Design review of the part built by this model. Coordinates are the model's own, in mm. A direction names the side the tool comes from. Coordinates: 2 decimals unless noted, no trailing zeros. Order: outer loops, then holes, each group sorted by start corner. A loop starts at its lowest first (then second) coordinate and runs counter-clockwise, first axis right, second up. Notation, with made-up numbers: M 0.5,-30 L 31.5,-30 A28 cw 31.5,0 Z; hole C 42.5,-18.75 d4. An arc over 180 degrees is marked long. Answer as a JSON object with one key per item and string values.
from build123d import *

# Parameters (mm, degrees)
BOSS_EXTRUDE1_DEPTH = 8
SKETCH2_R           = 1.75
CUT_EXTRUDE1_DEPTH  = 4


with BuildPart() as part:
    # Sketch1 → Boss-Extrude1 (new body)
    with BuildSketch(Plane.XY):
        with BuildLine():
            Line((-21, 0), (-12, 0))
            ThreePointArc((-12, 0), (-10.585786438, 0.585786438), (-10, 2))
            Line((-10, 2), (-10, 6.5))
            Line((-10, 6.5), (10, 6.5))
            Line((10, 6.5), (10, 2))
            ThreePointArc((10, 2), (10.585786438, 0.585786438), (12, 0))
            Line((12, 0), (21, 0))
            Line((21, 0), (21, 3))
            Line((21, 3), (13, 3))
            Line((13, 3), (13, 7.5))
            ThreePointArc((13, 7.5), (12.414213562, 8.914213562), (11, 9.5))
            Line((11, 9.5), (-11, 9.5))
            ThreePointArc((-11, 9.5), (-12.414213562, 8.914213562), (-13, 7.5))
            Line((-13, 7.5), (-13, 3))
            Line((-13, 3), (-21, 3))
            Line((-21, 3), (-21, 0))
        make_face()
    extrude(amount=BOSS_EXTRUDE1_DEPTH)

    # Sketch2 → Cut-Extrude1 (cut, through all)
    with BuildSketch(Plane(origin=(0, 3, 0), x_dir=(1, 0, 0), z_dir=(0, 1, 0))):
        with Locations((-17, -4)):
            Circle(SKETCH2_R)
        with Locations((17, -4)):
            Circle(SKETCH2_R)
    extrude(amount=-CUT_EXTRUDE1_DEPTH, mode=Mode.SUBTRACT)


solid = part.part
1) Tool access review of faces 5 (the flat face through (13, 5, 4)), 6 (the flat face through (-13, 5, 4)), 7 (the flat face through (0, 6.5, 4)): name each direction out of +Z, -Z, +X, -X, +Y, -Y from which nothing blocks a thin tool from reaching the whole face with its end or side.
Taken from the geometry:
{"face 5": "+Z, -Z, +X, +Y", "face 6": "+Z, -Z, -X, +Y", "face 7": "+Z, -Z, -Y"}
2) Add section B-B (y = 6). State the section outline as (x, z) points, and give its area (3 significant figures).
Taken from the geometry:
{"outline": "M -13,0 L -10,0 L -10,8 L -13,8 Z; M 10,0 L 13,0 L 13,8 L 10,8 Z", "area": "48.0 mm2"}
3) Add section C-C (x = -17). State the section outline as (y, z) points, and give its area (3 significant figures).
Taken from the geometry:
{"outline": "M 0,0 L 3,0 L 3,2.25 L 0,2.25 Z; M 0,5.75 L 3,5.75 L 3,8 L 0,8 Z", "area": "13.5 mm2"}
4) Add section A-A (y = 2.5). State the section outline as (x, z) points, and give its area (3 significant figures).
Taken from the geometry:
{"outline": "M -21,0 L -10,0 L -10,8 L -21,8 Z; M 10,0 L 21,0 L 21,8 L 10,8 Z; hole C -17,4 d3.5; hole C 17,4 d3.5", "area": "157 mm2"}
5) Mouldability with a two-part tool opening along X and no side actions: class faces 1 (the flat face through (10, 4, 4)), 2 (the flat face through (17, 3, 2)), 3 (the flat face through (-21, 2, 4)), 4 (the cylindrical face through (10.57, 0.6, 3.94)) as released by +X, released by -X, zero draft, split by the parting line, or undercut.
Taken from the geometry:
{"face 1": "undercut", "face 2": "zero draft", "face 3": "released by -X", "face 4": "undercut"}
6) To check wall thickness, follow L1, parallel to X at y = 5.25, z = 2.5; L2, parallel to X at y = 2.05, z = 4; L3, parallel to X at y = 0.7, z = 4. State the ranges of each line that lie inside material, in increasing order.
Taken from the geometry:
{"L1": "x = -13 to -10, 10 to 13", "L2": "x = -21 to -18.75, -15.25 to -10, 10 to 15.25, 18.75 to 21", "L3": "x = -21 to -18.75, -15.25 to -10.48, 10.48 to 15.25, 18.75 to 21"}
7) Add section D-D (z = 4). State the section outline as (x, y) points, and give its area (3 significant figures).
Taken from the geometry:
{"outline": "M -21,0 L -18.75,0 L -18.75,3 L -21,3 Z; M -15.25,0 L -12,0 A2 ccw -10,2 L -10,6.5 L 10,6.5 L 10,2 A2 ccw 12,0 L 15.25,0 L 15.25,3 L 13,3 L 13,7.5 A2 ccw 11,9.5 L -11,9.5 A2 ccw -13,7.5 L -13,3 L -15.25,3 Z; M 18.75,0 L 21,0 L 21,3 L 18.75,3 Z", "area": "141 mm2"}
8) Insertion check: pin 1 Ø4 at (x, z) = (-4, 4.5) entering from -Y; pin 2 Ø1.3 at (y, z) = (6, 5) entering from -X; pin 3 Ø4.5 at (x, z) = (17, 4) entering from +Y. Each pin has a flat end and moves straight along its axis. Give the tip position at first contact, or say it passes through.
Taken from the geometry:
{"pin 1": "stops at y = 6.5", "pin 2": "stops at x = -13", "pin 3": "stops at y = 3"}
